Design review of the part built by this model. Coordinates are the model's own, in mm. A direction names the side the tool comes from. Coordinates: 2 decimals unless noted, no trailing zeros. Loops run counter-clockwise (first coordinate to the right, second up) from the corner with the lowest first, then second, coordinate; pieces in that order, holes last. Notation, with made-up numbers: M 26,4 L 52,4 A16 cw 52,33 Z; hole C -24,17 d8. An arc over 180 degrees is marked long. Put each result on its own line as item: value. Start each with the question number.
(1) Take a section at D-D, the plane y = 83. Give the boundary of the cut face in (x, z), then the cut area to 3 significant figures.
(2) For probe 1 along X at (y, z) = (67.5, 226.5); probe 2 along X at (y, z) = (50, 125); probe 3 along Y at (x, z) = (38, 175), list the stretches that pass through material, from the lowest coordinate up. Write a range as [from, to].
(3) The part is to be moulded in two halves that separate along X. For faces 1 (the cylindrical face through (96.945, 97.103, 182.1)), 2 (the flat face through (10, 42.1, 189)), 3 (the flat face through (46, 98, 250)), say which applies: +X half, -X half, draft (parallel to the pull), parting line (faces both ways), or undercut.
(4) Clearance check with flat-ended pins moving along their axes: pin 1 (0.8 mm diameter, centred on x = 3, z = 234.5, fed in from -Y); pin 2 (7.5 mm diameter, centred on x = 92, z = 207, fed in from -Y); pin 3 (1 mm diameter, centred on x = 34, z = 224, fed in from -Y); pin 4 (2 mm diameter, centred on x = 98, z = 223, fed in from -Y). State where each tip first meets the part, or that it passes through.
(5) Take a section at A-A, the plane y = 50. Give the boundary of the cut face in (x, z).
(6) For faces 4 (the flat face through (98.75, 26, 230)), 5 (the flat face through (5, 50, 189)), 6 (the flat face through (94.5, 6, 232)), list the 3-axis set-ups (+Z, -Z, +X, -X, +Y, -Y) from which the entire face can be reached by the end or side of a thin tool; tool diameter is ignored.
(7) Take a section at B-B, the plane x = 50. Give the boundary of the cut face in (y, z).
```python
from build123d import *

# Parameters (mm, degrees)
SKETCH1_W                = 100
SKETCH1_H                = 100
BOSS_EXTRUDE1_DEPTH      = 250
SKETCH2_W                = 90
SKETCH2_H                = 90
CUT_EXTRUDE1_DEPTH       = 288.228132327
FILLET1_R                = 10.16
SKETCH3_W                = 9.3412
SKETCH3_H                = 5
BOSS_EXTRUDE2_DEPTH      = 250
SKETCH4_W                = 100
SKETCH4_H                = 125
CUT_EXTRUDE2_DEPTH       = 288.228132327
SKETCH6_W                = 90
SKETCH6_H                = 5.08
BOSS_EXTRUDE3_DEPTH      = 95
SKETCH7_R                = 45.3
CUT_EXTRUDE4_DEPTH       = 5.08
SKETCH10_R               = 48.300000047
BOSS_EXTRUDE4_DEPTH      = 30
SKETCH11_R               = 45.3
CUT_EXTRUDE5_DEPTH       = 30
SKETCH13_W               = 63.5
SKETCH13_H               = 63.5
CUT_EXTRUDE7_DEPTH       = 5
FILLET4_R                = 1.27
FILLET5_R                = 10.16
BOSS_EXTRUDE6_DEPTH      = 30
SKETCH16_R               = 45.3
CUT_EXTRUDE8_DEPTH       = 189.745860882
CUT_EXTRUDE10_DEPTH      = 210.821352584
SKETCH19_W               = 81
SKETCH19_H               = 64.77
CUT_EXTRUDE11_DEPTH      = 25.4
SKETCH20_W               = 81
SKETCH20_H               = 32.5
BOSS_EXTRUDE7_DEPTH      = 5
BOSS_EXTRUDE8_START      = 32.5
BOSS_EXTRUDE8_DEPTH      = 32.5
BOSS_EXTRUDE10_DEPTH     = 119.92
SKETCH25_W               = 73.5
SKETCH25_H               = 16.413635584
BOSS_EXTRUDE11_DEPTH     = 6.35
SKETCH26_W               = 17.272
SKETCH26_H               = 100
CUT_EXTRUDE12_DEPTH      = 132
SKETCH28_W               = 81
SKETCH28_H               = 37.9
CUT_EXTRUDE13_DEPTH      = 113.57
SKETCH29_W               = 2.5
SKETCH29_H               = 31.9
SKETCH29_H_2             = 27
CUT_EXTRUDE14_DEPTH      = 40
CUT_EXTRUDE15_DEPTH      = 198.405678703
CUT_EXTRUDE15_DEPTH_BACK = 119.92
SKETCH30_W               = 90
SKETCH30_H               = 37.9
BOSS_EXTRUDE12_DEPTH     = 119.92
CUT_EXTRUDE16_REACH      = 289.228
SKETCH33_W               = 89
SKETCH33_H               = 34.77
SKETCH35_W               = 4.5
SKETCH35_H               = 38.1
BOSS_EXTRUDE14_DEPTH     = 119.92


with BuildPart() as part:
    # Sketch1 → Boss-Extrude1 (new body)
    with BuildSketch(Plane.XY):
        with Locations((50, 50)):
            Rectangle(SKETCH1_W, SKETCH1_H)
    extrude(amount=BOSS_EXTRUDE1_DEPTH)

    # Sketch2 → Cut-Extrude1 (cut, through all)
    with BuildSketch(Plane(origin=(0, 0, 0), x_dir=(-1, 0, 0), z_dir=(0, 0, -1))):
        with Locations((-50, 50)):
            Rectangle(SKETCH2_W, SKETCH2_H)
    extrude(amount=-CUT_EXTRUDE1_DEPTH, mode=Mode.SUBTRACT)

    # Fillet1
    fillet1_edges = [part.edges().sort_by_distance(p)[0] for p in [
        (0, 100, 125),
        (0, 0, 125),
        (100, 0, 125),
        (100, 100, 125),
    ]]
    fillet(fillet1_edges, radius=FILLET1_R)

    # Sketch3 → Boss-Extrude2 (add, through all)
    with BuildSketch(Plane(origin=(0, 0, 0), x_dir=(-1, 0, 0), z_dir=(0, 0, -1))):
        with Locations((-90.3294, 55.4)):
            Rectangle(SKETCH3_W, SKETCH3_H)
        with Locations((-90.3294, 44.6)):
            Rectangle(SKETCH3_W, SKETCH3_H)
        with Locations((-9.6706, 44.6)):
            Rectangle(SKETCH3_W, SKETCH3_H)
        with Locations((-9.6706, 55.4)):
            Rectangle(SKETCH3_W, SKETCH3_H)
    extrude(amount=-BOSS_EXTRUDE2_DEPTH)

    # Sketch4 → Cut-Extrude2 (cut, through all)
    with BuildSketch(Plane(origin=(0, 100, 0), x_dir=(1, 0, 0), z_dir=(0, 1, 0))):
        with Locations((50, -62.5)):
            Rectangle(SKETCH4_W, SKETCH4_H)
    extrude(amount=-CUT_EXTRUDE2_DEPTH, mode=Mode.SUBTRACT)

    # Sketch6 → Boss-Extrude3 (add)
    with BuildSketch(Plane(origin=(0, 5, 0), x_dir=(1, 0, 0), z_dir=(0, 1, 0))):
        with Locations((50, -127.54)):
            Rectangle(SKETCH6_W, SKETCH6_H)
    extrude(amount=BOSS_EXTRUDE3_DEPTH)

    # Sketch7 → Cut-Extrude4 (cut)
    with BuildSketch(Plane(origin=(0, 0, 125), x_dir=(-1, 0, 0), z_dir=(0, 0, -1))):
        with Locations((-50, 50)):
            Circle(SKETCH7_R)
    extrude(amount=-CUT_EXTRUDE4_DEPTH, mode=Mode.SUBTRACT)

    # Sketch10 → Boss-Extrude4 (add)
    with BuildSketch(Plane(origin=(0, 0, 125), x_dir=(-1, 0, 0), z_dir=(0, 0, -1))):
        with Locations(Location((-50, 50, 0), (0, 0, 180))):
            Circle(SKETCH10_R)
    extrude(amount=BOSS_EXTRUDE4_DEPTH)

    # Sketch11 → Cut-Extrude5 (cut)
    with BuildSketch(Plane(origin=(0, 0, 95), x_dir=(-1, 0, 0), z_dir=(0, 0, -1))):
        with Locations((-50, 50)):
            Circle(SKETCH11_R)
    extrude(amount=-CUT_EXTRUDE5_DEPTH, mode=Mode.SUBTRACT)

    # Sketch13 → Cut-Extrude7 (cut)
    with BuildSketch(Plane.XZ):
        with Locations((50, 218.25)):
            Rectangle(SKETCH13_W, SKETCH13_H)
    extrude(amount=-CUT_EXTRUDE7_DEPTH, mode=Mode.SUBTRACT)

    # Fillet4
    fillet4_edges = [part.edges().sort_by_distance(p)[0] for p in [
        (81.75, 0, 218.25),
        (18.25, 0, 218.25),
        (50, 0, 186.5),
    ]]
    fillet(fillet4_edges, radius=FILLET4_R)

    # Fillet5
    fillet5_edges = [part.edges().sort_by_distance(p)[0] for p in [
        (95, 95, 190.04),
        (5, 95, 190.04),
        (5, 5, 190.04),
        (95, 5, 190.04),
    ]]
    fillet(fillet5_edges, radius=FILLET5_R)

    # Sketch14 → Boss-Extrude6 (add)
    with BuildSketch(Plane(origin=(0, 0, 125), x_dir=(-1, 0, 0), z_dir=(0, 0, -1))):
        with BuildLine():
            Line((-5, 100), (-95, 100))
            Line((-95, 100), (-95, 98.592142595))
            ThreePointArc((-95, 98.592142595), (-98.661881885, 94.879841267), (-100, 89.84))
            Line((-100, 89.84), (-100, 10.16))
            ThreePointArc((-100, 10.16), (-97.024204897, 2.975795103), (-89.84, 0))
            Line((-89.84, 0), (-10.16, 0))
            ThreePointArc((-10.16, 0), (-2.975795103, 2.975795103), (0, 10.16))
            Line((0, 10.16), (0, 89.84))
            ThreePointArc((0, 89.84), (-1.338118115, 94.879841267), (-5, 98.592142595))
            Line((-5, 98.592142595), (-5, 100))
        make_face()
    extrude(amount=BOSS_EXTRUDE6_DEPTH)

    # Sketch16 → Cut-Extrude8 (cut, through all)
    with BuildSketch(Plane.XY.offset(125)):
        with Locations(Location((50, 50, 0), (0, 0, 169.956667322))):
            Circle(SKETCH16_R)
    extrude(amount=-CUT_EXTRUDE8_DEPTH, mode=Mode.SUBTRACT)

    # Sketch18 → Cut-Extrude10 (cut, through all)
    with BuildSketch(Plane(origin=(0, 0, 95), x_dir=(-1, 0, 0), z_dir=(0, 0, -1))):
        with BuildLine():
            Line((-100, 89.84), (-100, 107.62))
            Line((-100, 107.62), (0, 107.62))
            Line((0, 107.62), (0, 89.84))
            ThreePointArc((0, 89.84), (-2.975795103, 97.024204897), (-10.16, 100))
            Line((-10.16, 100), (-89.84, 100))
            ThreePointArc((-89.84, 100), (-97.024204897, 97.024204897), (-100, 89.84))
        make_face()
    extrude(amount=-CUT_EXTRUDE10_DEPTH, mode=Mode.SUBTRACT)

    # Sketch19 → Cut-Extrude11 (cut)
    with BuildSketch(Plane.XZ):
        with Locations((50, 217.615)):
            Rectangle(SKETCH19_W, SKETCH19_H)
    extrude(amount=-CUT_EXTRUDE11_DEPTH, mode=Mode.SUBTRACT)

    # Sketch20 → Boss-Extrude7 (add)
    with BuildSketch(Plane.XZ):
        with Locations((50, 201.48)):
            Rectangle(SKETCH20_W, SKETCH20_H)
    extrude(amount=-BOSS_EXTRUDE7_DEPTH)

    # Sketch21 → Boss-Extrude8 (add)
    with BuildSketch(Plane.XY.offset(185.23).offset(BOSS_EXTRUDE8_START)):
        with BuildLine():
            Line((9.5, 5), (15.16, 5))
            ThreePointArc((15.16, 5), (12.201837845, 5.440181243), (9.5, 6.722583334))
            Line((9.5, 6.722583334), (9.5, 5))
        make_face()
        with BuildLine():
            ThreePointArc((90.5, 6.722583334), (87.798162155, 5.440181243), (84.84, 5))
            Line((84.84, 5), (90.5, 5))
            Line((90.5, 5), (90.5, 6.722583334))
        make_face()
    extrude(amount=-BOSS_EXTRUDE8_DEPTH)

    # Sketch24 → Boss-Extrude10 (add)
    with BuildSketch(Plane.XY.offset(130.08)):
        Polygon((95, 57.9), (86.75, 57.9), (86.75, 92.9), (13.25, 92.9), (13.25, 57.9), (5, 57.9), (5, 95), (95, 95), align=None)
    extrude(amount=BOSS_EXTRUDE10_DEPTH)

    # Sketch25 → Boss-Extrude11 (add)
    with BuildSketch(Plane.XY.offset(130.08)):
        with Locations((50, 84.693182208)):
            Rectangle(SKETCH25_W, SKETCH25_H)
    extrude(amount=BOSS_EXTRUDE11_DEPTH)

    # Sketch26 → Cut-Extrude12 (cut)
    with BuildSketch(Plane.ZY):
        with Locations((103.636, 50)):
            Rectangle(SKETCH26_W, SKETCH26_H)
    extrude(amount=-CUT_EXTRUDE12_DEPTH, mode=Mode.SUBTRACT)

    # Sketch28 → Cut-Extrude13 (cut)
    with BuildSketch(Plane.XY.offset(250)):
        with Locations((50, 76.85)):
            Rectangle(SKETCH28_W, SKETCH28_H)
    extrude(amount=-CUT_EXTRUDE13_DEPTH, mode=Mode.SUBTRACT)

    # Sketch29 → Cut-Extrude14 (cut)
    with BuildSketch(Plane.XY.offset(250)):
        with Locations((2.5, 73.85)):
            Rectangle(SKETCH29_W, SKETCH29_H)
        with Locations((2.5, 26.1)):
            Rectangle(SKETCH29_W, SKETCH29_H_2)
        with Locations((97.5, 26.1)):
            Rectangle(SKETCH29_W, SKETCH29_H_2)
        with Locations((97.5, 73.85)):
            Rectangle(SKETCH29_W, SKETCH29_H)
    extrude(amount=-CUT_EXTRUDE14_DEPTH, mode=Mode.SUBTRACT)

    # Sketch30 → Cut-Extrude15 (cut, two sides: drawn at the far end of the back side and taken through both)
    with BuildSketch(Plane.XY.offset(250).offset(-CUT_EXTRUDE15_DEPTH_BACK)):
        with Locations((50, 76.85)):
            Rectangle(SKETCH30_W, SKETCH30_H)
    extrude(amount=CUT_EXTRUDE15_DEPTH + CUT_EXTRUDE15_DEPTH_BACK, mode=Mode.SUBTRACT)

    # Sketch32 → Boss-Extrude12 (add)
    with BuildSketch(Plane.XY.offset(130.08)):
        with BuildLine():
            Line((15.16, 95), (84.84, 95))
            ThreePointArc((84.84, 95), (92.024204897, 92.024204897), (95, 84.84))
            Line((95, 84.84), (95, 95.8))
            Line((95, 95.8), (5, 95.8))
            Line((5, 95.8), (5, 84.84))
            ThreePointArc((5, 84.84), (7.975795103, 92.024204897), (15.16, 95))
        make_face()
    extrude(amount=BOSS_EXTRUDE12_DEPTH)

    # Cut-Extrude16: up to this face of the body (flat: up to its plane)
    cut_extrude16_end = Plane(part.part.faces().sort_by_distance((9.6706, 42.1, 190.04))[0])
    # Sketch33 → Cut-Extrude16 (cut, up to the picked face)
    with BuildSketch(Plane.XZ, mode=Mode.PRIVATE) as cut_extrude16_sk1:
        with Locations((50, 232.615)):
            Rectangle(SKETCH33_W, SKETCH33_H)
    cut_extrude16_tool1 = split(extrude(cut_extrude16_sk1.sketch, amount=-CUT_EXTRUDE16_REACH, mode=Mode.PRIVATE), bisect_by=cut_extrude16_end, keep=Keep.BOTH, mode=Mode.PRIVATE)
    add(cut_extrude16_tool1.solids().sort_by(Axis((50, 0, 232.615), (0, 1, 0)))[0], mode=Mode.SUBTRACT)

    # Sketch35 → Boss-Extrude14 (add)
    with BuildSketch(Plane.XY.offset(250)):
        with Locations((7.25, 76.95)):
            Rectangle(SKETCH35_W, SKETCH35_H)
        with Locations((92.75, 76.95)):
            Rectangle(SKETCH35_W, SKETCH35_H)
    extrude(amount=-BOSS_EXTRUDE14_DEPTH)


solid = part.part
```
Computed values:
1. outline: M 0,112.27 L 18.97,112.27 L 18.97,130.08 L 9.5,130.08 L 9.5,250 L 3.75,250 L 3.75,210 L 1.25,210 L 1.25,250 L 0,250 Z; M 81.03,112.27 L 100,112.27 L 100,250 L 98.75,250 L 98.75,210 L 96.25,210 L 96.25,250 L 90.5,250 L 90.5,130.08 L 81.03,130.08 Z
1. area: 2,750 mm^2
2. probe 1: x = [0, 1.25], [3.75, 9.5], [90.5, 96.25], [98.75, 100]
2. probe 2: x = [0, 4.7], [95.3, 100]
2. probe 3: y = [0, 5], [95, 100]
3. face 1: +X half
3. face 2: undercut
3. face 3: draft
4. pin 1: stops at y = 2.58
4. pin 2: stops at y = 0
4. pin 3: stops at y = 95
4. pin 4: stops at y = 2.95
5. outline: M 0,112.27 L 4.7,112.27 L 4.7,130.08 L 5,130.08 L 5,250 L 0,250 Z; M 95,130.08 L 95.3,130.08 L 95.3,112.27 L 100,112.27 L 100,250 L 95,250 Z
6. face 4: +Z
6. face 5: +Z, -Z
6. face 6: +Z, -Y
7. outline: M 0,112.27 L 4.7,112.27 L 4.7,130.08 L 5,130.08 L 5,215.23 L 0,215.23 Z; M 95,130.08 L 95.3,130.08 L 95.3,112.27 L 100,112.27 L 100,250 L 95,250 Z
